Print and shaded views of the part. All mm, measured from the part's lowest x, y and z. A direction names the side the tool comes from. Coordinates: 2 decimals unless noted, no trailing zeros. Loops run counter-clockwise (first coordinate to the right, second up) from the corner with the lowest first, then second, coordinate; pieces in that order, holes last.
1) Saw through at A-A, the plane y = 4.6. Write the cut outline in (x, z).
2) Saw through at C-C, the plane z = 5.5. Write the cut outline in (x, y).
3) Saw through at B-B, the plane x = 14. Write the cut outline in (y, z).
4) Which spindle directions (+Z, -Z, +X, -X, +Y, -Y) get a long thin tool onto all of the face, cutting with end or side? Do the marked faces 1 and 2. Say none if no direction does.
5) Pin check, flat tips, straight feed: pin 1 Ø1.5 at (x, y) = (8.5, 0.5) entering from -Z; pin 2 Ø2.5 at (y, z) = (1.5, 28.5) entering from +X; pin 3 Ø1.6 at (y, z) = (2.5, 16.5) entering from +X; pin 4 Ø8 at (x, z) = (11, 7.5) entering from -Y. Stop position of each tip, or through.
6) Wall check: line 1 along Z through (x, y) = (26, 4.6); line 2 along X through (y, z) = (0.6, 7.5). Give the ranges that are in metal, low to high.
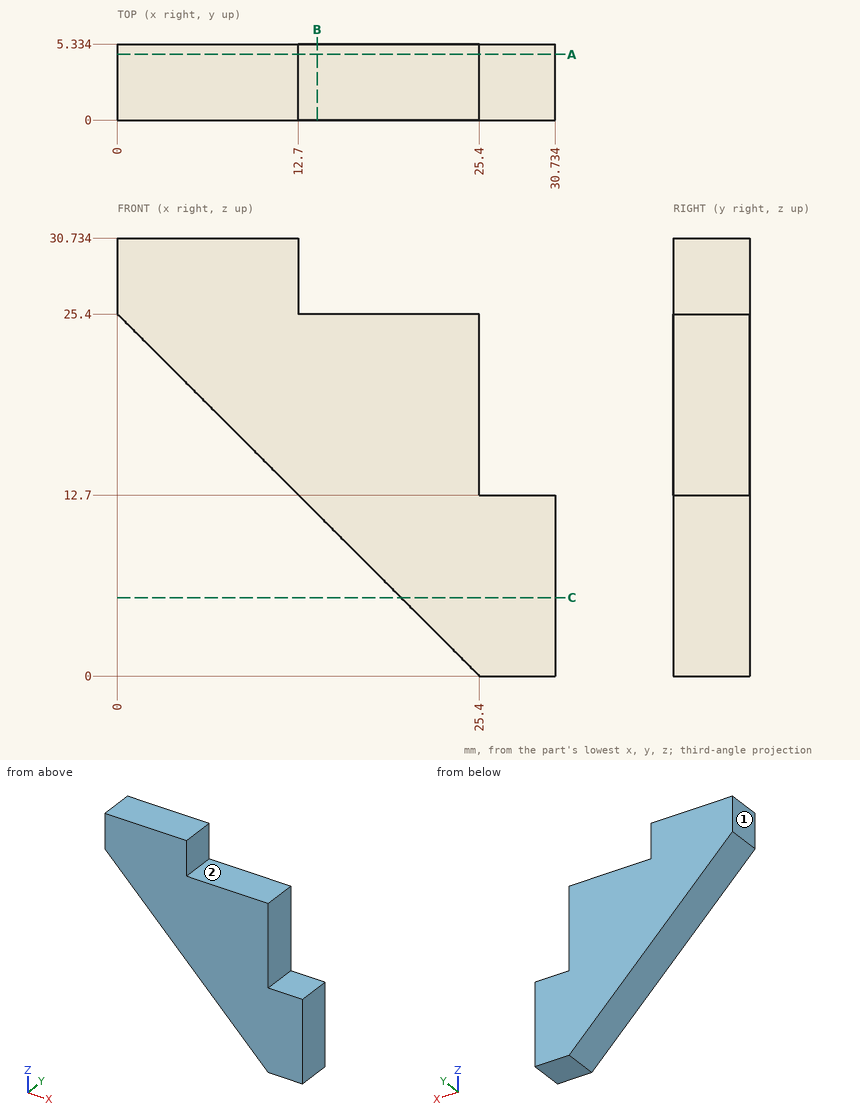
Data:
1. outline: (0, 25.4) - (25.4, 0) - (30.73, 0) - (30.73, 12.7) - (25.4, 12.7) - (25.4, 25.4) - (12.7, 25.4) - (12.7, 30.73) - (0, 30.73) - close
2. outline: (19.9, 0) - (30.73, 0) - (30.73, 5.33) - (19.9, 5.33) - close
3. outline: (0, 11.4) - (5.33, 11.4) - (5.33, 25.4) - (0, 25.4) - close
4. face 1: +Z, -Z, -X, +Y, -Y
4. face 2: +Z, +X, +Y, -Y
5. pin 1: stops at z = 16.15
5. pin 2: stops at x = 12.7
5. pin 3: stops at x = 25.4
5. pin 4: passes through
6. line 1: z = 0 to 12.7
6. line 2: x = 17.9 to 30.73
